Input: part model. Units: mm. Frame: model coordinates. A direction names the side the tool comes from. Coordinates: 2 decimals unless noted, no trailing zeros. Loops run counter-clockwise (first coordinate to the right, second up) from the corner with the lowest first, then second, coordinate; pieces in that order, holes last.
(1) Contact query for flat-ended pins moving along their axis: P1, Ø4, axis at y = 0.5, z = 26, coming from the -X side (3 decimals); P2, Ø5, axis at x = 2, z = 30.5, coming from the -Y side (3 decimals); P3, Ø1, axis at y = -3, z = 34, coming from the -X side. Output: stop coordinate, or through.
(2) Section A-A, the plane x = 0. Return loops of the section in (y, z) (3 decimals).
(3) Set-up query: faces 1 (the face through (2, -3, 0)), 2 (the face through (2, 0, 38.1)), 3 (the face through (0, 0, 27.94)). Return all of +Z, -Z, +X, -X, +Y, -Y with unobstructed straight access to the full face (end or side cutting, diameter ignored); none if empty.
(4) Section C-C, the plane z = 32. Return loops of the section in (x, y) (3 decimals).
(5) Mould query, pull axis X, two halves, no side actions, for faces 4 (the face through (-1.974, 0.068, 33.091)), 5 (the face through (0, 0, -2.54)), 6 (the face through (-0.96, -4.34, 36.81)). Classes: released by +X, released by -X, zero draft, split by the parting line, or undercut.
(6) Section D-D, the plane z = 7.5. Return loops of the section in (x, y) (3 decimals), then the cut area to 3 significant figures.
(7) Section B-B, the plane y = 3.75. Return loops of the section in (x, z), then the cut area to 3 significant figures.
(8) Line query: L1, parallel to Z at x = -2, y = -2.5; L2, parallel to Y at x = 0, z = 33 (3 decimals); L3, parallel to X at y = -1, z = 31.5 (3 decimals). Output: solid intervals per line, ascending.
```python
from build123d import *

# Parameters (mm, degrees)
SKETCH1_R           = 3.175
BOSS_EXTRUDE1_DEPTH = 35.56
SKETCH3_R           = 4.445
BOSS_EXTRUDE2_DEPTH = 2.54
CUT_EXTRUDE1_DEPTH  = 10.16


with BuildPart() as part:
    # Sketch1 → Boss-Extrude1 (new body)
    with BuildSketch(Plane.XY):
        Circle(SKETCH1_R)
    extrude(amount=BOSS_EXTRUDE1_DEPTH)

    # Sketch3 → Boss-Extrude2 (add)
    with BuildSketch(Plane.XY.offset(35.56)):
        Circle(SKETCH3_R)
    boss_extrude2 = extrude(amount=BOSS_EXTRUDE2_DEPTH)

    # Mirror1: Boss-Extrude2 across plane
    add(boss_extrude2.mirror(Plane.XY.offset(17.78)))

    # Sketch4 → Cut-Extrude1 (cut)
    with BuildSketch(Plane.XY.offset(38.1)):
        with BuildLine():
            Line((1.525, 0), (1.525, 1.25499004))
            ThreePointArc((1.525, 1.25499004), (-1.975, 0), (1.525, -1.25499004))
            Line((1.525, -1.25499004), (1.525, 0))
        make_face()
    extrude(amount=-CUT_EXTRUDE1_DEPTH, mode=Mode.SUBTRACT)


solid = part.part
```
Report:
1. P1: stops at x = -3.175
1. P2: stops at y = -3.175
1. P3: stops at x = -1.96
2. outline: (-4.445, -2.54) - (4.445, -2.54) - (4.445, 0) - (3.175, 0) - (3.175, 35.56) - (4.445, 35.56) - (4.445, 38.1) - (1.975, 38.1) - (1.975, 27.94) - (-1.975, 27.94) - (-1.975, 38.1) - (-4.445, 38.1) - (-4.445, 35.56) - (-3.175, 35.56) - (-3.175, 0) - (-4.445, 0) - close
3. face 1: none
3. face 2: +Z, +X, -X, +Y, -Y
3. face 3: +Z
4. outline: circle Ø6.35 at (0, 0); hole (1.525, -1.255) - (1.525, 1.255) arc R1.975 ccw (long way) to start
5. face 4: undercut
5. face 5: zero draft
5. face 6: split by the parting line
6. outline: circle Ø6.35 at (0, 0)
6. area: 31.7 mm2
7. outline: (-2.39, -2.54) - (2.39, -2.54) - (2.39, 0) - (-2.39, 0) - close; (-2.39, 35.56) - (2.39, 35.56) - (2.39, 38.1) - (-2.39, 38.1) - close
7. area: 24.2 mm2
8. L1: z = -2.54 to 0, 35.56 to 38.1
8. L2: y = -3.175 to -1.975, 1.975 to 3.175
8. L3: x = -3.013 to -1.703, 1.525 to 3.013
